Autodesk Inventor part; units mm, degrees
ref_plane "Work Plane1" through (10, 0, 42.5) normal (0, 0, -1) x (-1, 0, 0)
ref_plane "Work Plane2" through (0, 0, 22.5) normal (0, 0, 1) x (1, 0, 0)
ref_plane "YZ Plane" through (0, 0, 0) normal (1, 0, 0) x (0, 1, 0)
sketch "Sketch1" plane through (0, 0, 0) normal (0, 1, 0) x (-1, 0, 0)
  line L0 (0, 0) -> (-5, 0)
  line L1 (-5, 0) -> (-5, 45)
  line L2 (-5, 45) -> (0, 45)
  line L3 (0, 45) -> (0, 0)
  line L4 (-5, 45) -> (-20, 45)
  line L5 (-20, 45) -> (-20, 40)
  line L6 (-20, 40) -> (-5, 40)
  line L7 (-5, 40) -> (-5, 45)
  line L8 (-5, 0) -> (-20, 0)
  line L9 (-20, 0) -> (-20, 5)
  line L10 (-20, 5) -> (-5, 5)
  line L11 (-5, 5) -> (-5, 0)
  point P0 (-5, 40)
  point P1 (-5, 5)
  dimension "d0" = 5
  dimension "d1" = 5
  dimension "d2" = 5
  dimension "d3" = 15
  dimension "d4" = 15
  dimension "d5" = 35
extrude "Extrusion1" add sketch "Sketch1" along normal blind 20
sketch "Sketch2" plane through (0, 0, 45) normal (0, 0, 1) x (1, 0, 0)
  circle A0 centre (10, 10) radius 1.75
  line L0 (20, 0) -> (20, 20)
  line L1 (20, 0) -> (10, 0)
  line L2 (10, 0) -> (10, 20)
  line L3 (10, 20) -> (20, 20)
  line L4 (20, 20) -> (20, 0)
  line L5 (0, 0) -> (20, 0)
  dimension "d8" = 10
  dimension "d9" = 10
  dimension "d10" = 10
  dimension "d11" = 3.5
extrude "Extrusion2" cut sketch "Sketch2" against normal blind 200
sketch "Sketch3" plane through (0, 0, 0) normal (-1, 0, 0) x (0, 0, 1)
  line L0 (5, 0) -> (5, 20)
  line L1 (40, 0) -> (40, 20)
  line L2 (5, 15) -> (40, 15)
  line L3 (40, 15) -> (40, 5)
  line L4 (40, 5) -> (5, 5)
  line L5 (5, 5) -> (5, 15)
  line L6 (0, 20) -> (45, 20)
  line L7 (0, 0) -> (45, 0)
  point P0 (5, 5)
  dimension "d14" = 5
  dimension "d15" = 5
extrude "Extrusion3" cut sketch "Sketch3" against normal blind 20 contours L0 L2 L1 L4
sketch "Sketch4" plane through (0, 0, 0) normal (-1, 0, 0) x (0, 0, 1)
  line L0 (45, 0) -> (45, 20)
  line L1 (45, 20) -> (55, 20)
  line L2 (55, 20) -> (55, 0)
  line L3 (55, 0) -> (45, 0)
  line L4 (45, 0) -> (45, 20)
  line L5 (0, 20) -> (0, 11.75)
  line L6 (0, 20) -> (-10, 20)
  line L7 (-10, 20) -> (-10, 0)
  line L8 (-10, 0) -> (0, 0)
  line L9 (0, 0) -> (0, 20)
  circle A0 centre (50, 3) radius 1.375
  circle A1 centre (50, 17) radius 1.375
  circle A2 centre (-5, 17) radius 1.375
  circle A3 centre (-5, 3) radius 1.375
  point P0 (0, 0)
  point P1 (50, 20)
  dimension "d18" = 10
  dimension "d19" = 10
  dimension "d20" = 3
  dimension "d21" = 3
  dimension "d22" = 5
  dimension "d23" = 5
  dimension "d24" = 5
  dimension "d25" = 5
  dimension "d26" = 3
  dimension "d27" = 3
  dimension "d28" = 2.75
  dimension "d29" = 2.75
  dimension "d30" = 2.75
  dimension "d31" = 2.75
extrude "Extrusion4" add sketch "Sketch4" against normal blind 5
sketch "Sketch5" plane through (10, 11.75, 45) normal (1, 0, 0) x (0, 0, -1)
  circle A0 centre (42.5, 5.75) radius 1.35
  circle A1 centre (42.5, -9.25) radius 1.35
  circle A2 centre (2.5, 5.75) radius 1.35
  circle A3 centre (2.5, -9.25) radius 1.35
  line L0 (40, 8.25) -> (45, 8.25)
  line L1 (45, 8.25) -> (45, 0)
  line L2 (45, -3.5) -> (45, -11.75)
  line L3 (45, -11.75) -> (40, -11.75)
  line L4 (5, -11.75) -> (0, -11.75)
  line L5 (0, -11.75) -> (0, -3.5)
  line L6 (0, 0) -> (0, 8.25)
  line L7 (0, 8.25) -> (5, 8.25)
  dimension "d34" = 2.5
  dimension "d35" = 2.5
  dimension "d36" = 2.5
  dimension "d37" = 2.5
  dimension "d38" = 2.5
  dimension "d39" = 2.5
  dimension "d40" = 2.5
  dimension "d41" = 2.5
  dimension "d42" = 2.7
  dimension "d43" = 2.7
  dimension "d44" = 2.7
  dimension "d45" = 2.7
extrude "Extrusion5" cut sketch "Sketch5" against normal blind 15
sketch "Sketch6" plane through (0, 0, 55) normal (-1, 0, 0) x (0, 0, 1)
  circle A0 centre (-12.5, 17.5) radius 1.35
  circle A1 centre (-12.5, 17.5) radius 2.35
  circle A2 centre (-12.5, 2.5) radius 1.35
  circle A3 centre (-12.5, 2.5) radius 2.35
  circle A4 centre (-52.5, 2.5) radius 1.35
  circle A5 centre (-52.5, 2.5) radius 2.35
  circle A6 centre (-52.5, 17.5) radius 1.35
  circle A7 centre (-52.5, 17.5) radius 2.35
  point P0 (-55, 0)
  dimension "d48" = 4.7
  dimension "d49" = 4.7
  dimension "d50" = 4.7
  dimension "d51" = 4.7
extrude "Extrusion6" cut sketch "Sketch6" against normal blind 7.5 contours A0 | A1 | A2 | A3 | A4 | A5 | A6 | A7
ref_plane "Work Plane1" through (10, 0, 42.5) normal (0, 0, -1) x (-1, 0, 0)
sketch "Sketch7" plane through (10, 0, 42.5) normal (0, 0, -1) x (-1, 0, 0)
  line L0 (0, 11.75) -> (0, 20)
  line L1 (5, 20) -> (0, 20)
  line L2 (5, 0) -> (0, 0)
  arc A0 (0, 8.25) -> (0, 11.75) centre (0, 10) ccw
  line L3 (0, 20) -> (0, 11.75)
  line L4 (0, 13.1754) -> (2.75, 11.5877)
  line L5 (2.75, 11.5877) -> (2.75, 8.4123)
  line L6 (2.75, 8.4123) -> (0, 6.8246)
  line L7 (0, 6.8246) -> (-2.75, 8.4123)
  line L8 (-2.75, 8.4123) -> (-2.75, 11.5877)
  line L9 (-2.75, 11.5877) -> (0, 13.1754)
  point P0 (10, 0)
  dimension "d57" = 20
  dimension "d60" = 2.75
extrude "Extrusion7" cut sketch "Sketch7" along normal mid plane 2.4
ref_plane "Work Plane2" through (0, 0, 22.5) normal (0, 0, 1) x (1, 0, 0)
mirror "Mirror1" about plane through (0, 0, 22.5) normal (0, 0, 1) of "Extrusion7"
equation "\"d14\" = d15"
equation "\"d19\" = d18"
equation "\"d20\" = d21"
equation "\"d24\" = d23"
equation "\"d25\" = d22"
equation "\"d26\" = d20"
equation "\"d27\" = d21"
equation "\"d34\" = d35"
equation "\"d37\" = d34"
equation "\"d38\" = d34"
equation "\"d39\" = d36"
equation "\"d40\" = d39"
equation "\"d41\" = d34"
equation "\"d43\" = d42"
equation "\"d44\" = d42"
equation "\"d45\" = d43"
equation "\"d49\" = d48"
equation "\"d50\" = d49"
equation "\"d51\" = d48"
properties part number "MotorDifferentialMountingBracket" material "Stainless Steel"
Geometry check sheet. Reference: the model listing, model coordinates, mm. A direction names the side the tool comes from. Give positions to 0.01 mm unless a question says otherwise; leave off trailing zeros. Write each loop counter-clockwise with the first axis right and the second up, starting at its lowest first coordinate (ties: lowest second). Pieces come first, ordered by that corner, then holes.
1) Section check D-D, the plane x = 2.75. State how many separate pieces and enclosed holes the cut face has, and give its area (3 significant figures).
2) Section check B-B, the plane x = 5.75. Record the boundary of the cut face in (y, z), and give its area (3 significant figures).
3) Section check A-A, the plane z = 29. Record the boundary of the cut face in (x, y).
4) Gauge pin test, flat ends, axial feed: pin 1 (4.5 mm diameter, centred on y = 2.5, z = 2.5, fed in from -X); pin 2 (4 mm diameter, centred on y = 17.5, z = 16, fed in from +X); pin 3 (4 mm diameter, centred on x = 7.5, y = 18, fed in from +Z). Record the tip position at first contact, or that the pin passes through.
5) Material ranges on L1, parallel to Y at x = 1.2, z = 50 (3 decimals); L2, parallel to Z at x = 7.5, y = 10.25; L3, parallel to Y at x = 5, z = 2.5, recorded low to high.
6) Release check for a two-part mould opening along Y. For faces 1 (the cylindrical face through (2.465, 3.06, 48.626)), 2 (the flat face through (8, 10, 41.3)), 3 (the flat face through (3, 20, 23)), 4 (the flat face through (5, 17, 22)) record: pulls with the +Y half, pulls with the -Y half, needs draft (parallel to the pull), parting line crosses it, or undercut.
7) Section check C-C, the plane y = 10. Record the boundary of the cut face in (x, z).
8) Access from +Z, -Z, +X, -X, +Y, -Y to the whole of each face (thin tool, end or side, straight path). Record for faces 5 (the flat face through (7.5, 16, 4)), 6 (the flat face through (8, 10, 43.7)), 7 (the flat face through (5, 2, 22)).
Computed:
1. separate pieces: 1
1. enclosed holes: 9
1. area: 857 mm2
2. outline: (0, 0) - (20, 0) - (20, 5) - (0, 5) - close; (0, 40) - (20, 40) - (20, 45) - (0, 45) - close; hole circle Ø4.7 at (2.5, 2.5); hole circle Ø4.7 at (2.5, 42.5); hole circle Ø4.7 at (17.5, 2.5); hole circle Ø4.7 at (17.5, 42.5)
2. area: 131 mm2
3. outline: (0, 0) - (5, 0) - (5, 5) - (0, 5) - close; (0, 15) - (5, 15) - (5, 20) - (0, 20) - close
4. pin 1: stops at x = 7.5
4. pin 2: stops at x = 5
4. pin 3: stops at z = 45
5. L1: y = 0 to 1.625, 4.375 to 15.625, 18.375 to 20
5. L2: z = 0 to 1.3, 3.7 to 5, 40 to 41.3, 43.7 to 45
5. L3: y = 0 to 0.15, 4.85 to 15.15, 19.85 to 20
6. face 1: undercut
6. face 2: undercut
6. face 3: pulls with the +Y half
6. face 4: needs draft
7. outline: (0, -10) - (5, -10) - (5, 0) - (8.25, 0) - (8.25, 1.3) - (7.25, 1.3) - (7.25, 3.7) - (8.25, 3.7) - (8.25, 5) - (0, 5) - close; (0, 40) - (8.25, 40) - (8.25, 41.3) - (7.25, 41.3) - (7.25, 43.7) - (8.25, 43.7) - (8.25, 45) - (5, 45) - (5, 55) - (0, 55) - close
8. face 5: -X
8. face 6: +X
8. face 7: +X, +Y, -Y
